```python
from build123d import *
from build123d.topology import SkipClean

# Parameters (mm, degrees)
SKETCH1_W             = 80
SKETCH1_H             = 80
BOSS_EXTRUDE1_DEPTH   = 1.5
FILLET1_R             = 4
BOSS_EXTRUDE2_START   = 1.5
SKETCH2_R             = 4
BOSS_EXTRUDE2_DEPTH   = 1.5
F_4_0MM_DOWEL_HOLE1_D = 4
CUT_EXTRUDE1_DEPTH    = 1.5


with BuildPart() as part:
    # Sketch1 → Boss-Extrude1 (new body)
    with BuildSketch(Plane.XY):
        with Locations((40, 40)):
            Rectangle(SKETCH1_W, SKETCH1_H)
    extrude(amount=BOSS_EXTRUDE1_DEPTH)

    # Fillet1
    fillet1_edges = [part.edges().sort_by_distance(p)[0] for p in [
        (0, 0, 0.75),
        (0, 80, 0.75),
        (80, 80, 0.75),
        (80, 0, 0.75),
    ]]
    fillet(fillet1_edges, radius=FILLET1_R)

    # Sketch2 → Boss-Extrude2 (add)
    with SkipClean():  # the faces are left unmerged after this step: merging them gives an invalid solid
        with BuildSketch(Plane.XY.offset(1.5).offset(BOSS_EXTRUDE2_START)):
            with Locations(Location((4, 76, 0), (0, 0, 180))):
                Circle(SKETCH2_R)
            with Locations((76, 76)):
                Circle(SKETCH2_R)
            with Locations((4, 4)):
                Circle(SKETCH2_R)
            with Locations((76, 4)):
                Circle(SKETCH2_R)
        extrude(amount=-BOSS_EXTRUDE2_DEPTH)

    # 4.0mm Dowel Hole1 (through all)
    with Locations(Plane(origin=(0, 0, 0), x_dir=(-1, 0, 0), z_dir=(0, 0, -1))):
        with Locations((-4, 4), (-76, 4), (-76, 76), (-4, 76)):
            Hole(F_4_0MM_DOWEL_HOLE1_D / 2)

    # Sketch5 → Cut-Extrude1 (cut)
    with SkipClean():  # the faces are left unmerged after this step: merging them gives an invalid solid
        with BuildSketch(Plane(origin=(0, 0, 0), x_dir=(-1, 0, 0), z_dir=(0, 0, -1))):
            with BuildLine():
                Line((-55.934284639, 54.434284639), (-71, 69.5))
                Line((-71, 69.5), (-71, 10.5))
                Line((-71, 10.5), (-55.934284639, 25.565715361))
                ThreePointArc((-55.934284639, 25.565715361), (-61.5, 40), (-55.934284639, 54.434284639))
            make_face()
            with BuildLine():
                Line((-41.5, 40), (-54.164078425, 52.664078425))
                ThreePointArc((-54.164078425, 52.664078425), (-59, 40), (-54.164078425, 27.335921575))
                Line((-54.164078425, 27.335921575), (-41.5, 40))
            make_face()
            with BuildLine():
                Line((-40, 41.5), (-27.335921575, 54.164078425))
                ThreePointArc((-27.335921575, 54.164078425), (-40, 59), (-52.664078425, 54.164078425))
                Line((-52.664078425, 54.164078425), (-40, 41.5))
            make_face()
            with BuildLine():
                Line((-10.5, 71), (-69.5, 71))
                Line((-69.5, 71), (-54.434284639, 55.934284639))
                ThreePointArc((-54.434284639, 55.934284639), (-40, 61.5), (-25.565715361, 55.934284639))
                Line((-25.565715361, 55.934284639), (-10.5, 71))
            make_face()
            with BuildLine():
                Line((-9, 10.5), (-9, 69.5))
                Line((-9, 69.5), (-24.065715361, 54.434284639))
                ThreePointArc((-24.065715361, 54.434284639), (-18.5, 40), (-24.065715361, 25.565715361))
                Line((-24.065715361, 25.565715361), (-9, 10.5))
            make_face()
            with BuildLine():
                Line((-25.835921575, 27.335921575), (-38.5, 40))
                Line((-38.5, 40), (-25.835921575, 52.664078425))
                ThreePointArc((-25.835921575, 52.664078425), (-21, 40), (-25.835921575, 27.335921575))
            make_face()
            with BuildLine():
                Line((-52.664078425, 25.835921575), (-40, 38.5))
                Line((-40, 38.5), (-27.335921575, 25.835921575))
                ThreePointArc((-27.335921575, 25.835921575), (-40, 21), (-52.664078425, 25.835921575))
            make_face()
            with BuildLine():
                Line((-54.434284639, 24.065715361), (-69.5, 9))
                Line((-69.5, 9), (-10.5, 9))
                Line((-10.5, 9), (-25.565715361, 24.065715361))
                ThreePointArc((-25.565715361, 24.065715361), (-40, 18.5), (-54.434284639, 24.065715361))
            make_face()
        extrude(amount=-CUT_EXTRUDE1_DEPTH, mode=Mode.SUBTRACT)
    add(part.part.scale(1), mode=Mode.REPLACE)  # the faces are merged on a copy


solid = part.part
```
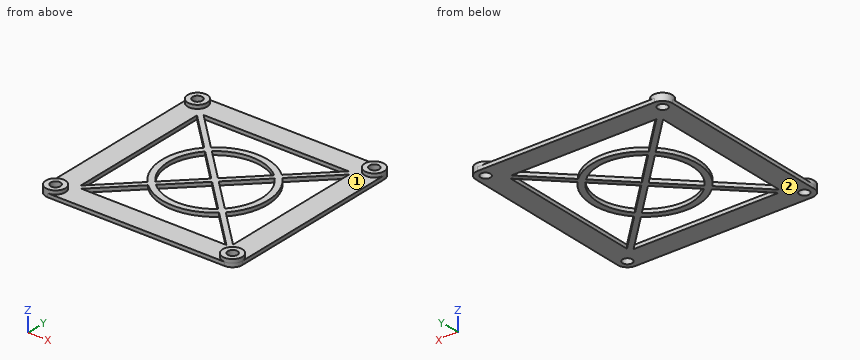
Geometry: final body of the model. Coordinates: model frame, mm. Face numbers are marked on the shaded views. Coordinates: 2 decimals unless noted, no trailing zeros. Write each loop counter-clockwise with the first axis right and the second up, starting at its lowest first coordinate (ties: lowest second). Pieces come first, ordered by that corner, then holes. Notation, with made-up numbers: M 55,69.25 L 89,69.25 A15 ccw 89,82.25 Z; hole C -6.5,86 d4. An arc over 180 degrees is marked long. Use CSV: the item, a comma, the result in double quotes. Start each with the question number.
1. First-contact query: P1, Ø24, axis at x = 26, y = 23.5, coming from the +Z side. Flat tip, straight axial feed; report the tip coordinate or a pass-through.
2. Ray query, probe 1 along Y at (x, z) = (4, 2.1); probe 2 along Y at (x, z) = (74.5, 0.45); probe 3 along Y at (x, z) = (76, 0.95). Return the intervals inside material, ascending.
3. Cut plane B-B on y = 64.5. Return the cut outline in (x, z), plus the area to 3 significant figures.
4. Cut plane D-D on x = 44.5. Return the cut outline in (y, z).
5. Mould query, pull axis Y, two halves, no side actions, for the marked faces 1 and 2. Classes: pulls with the +Y half, pulls with the -Y half, needs draft (parallel to the pull), parting line crosses it, or undercut.
6. Cut plane A-A on x = 66.5. Return the cut outline in (y, z).
7. Cut plane C-C on z = 0.6. Count the separate pieces of the cut face and the enclosed holes in it, plus the area to 3 significant figures.
Entries:
1,P1,"z = 1.5"
2,probe 1,"0 to 2, 6 to 8, 72 to 74, 78 to 80"
2,probe 2,"0 to 2.68, 5.32 to 74.68, 77.32 to 80"
2,probe 3,"0 to 2, 6 to 74, 78 to 80"
3,outline,"M 0,0 L 9,0 L 9,1.5 L 0,1.5 Z; M 14,0 L 17,0 L 17,1.5 L 14,1.5 Z; M 63,0 L 66,0 L 66,1.5 L 63,1.5 Z; M 71,0 L 80,0 L 80,1.5 L 71,1.5 Z"
3,area,"36.0 mm²"
4,outline,"M 0,0 L 9,0 L 9,1.5 L 0,1.5 Z; M 18.98,0 L 21.54,0 L 21.54,1.5 L 18.98,1.5 Z; M 34,0 L 37,0 L 37,1.5 L 34,1.5 Z; M 43,0 L 46,0 L 46,1.5 L 43,1.5 Z; M 58.46,0 L 61.02,0 L 61.02,1.5 L 58.46,1.5 Z; M 71,0 L 80,0 L 80,1.5 L 71,1.5 Z"
5,face 1,"undercut"
5,face 2,"needs draft"
6,outline,"M 0,0 L 9,0 L 9,1.5 L 0,1.5 Z; M 12,0 L 15,0 L 15,1.5 L 12,1.5 Z; M 65,0 L 68,0 L 68,1.5 L 65,1.5 Z; M 71,0 L 80,0 L 80,1.5 L 71,1.5 Z"
7,separate pieces,"1"
7,enclosed holes,"12"
7,area,"3,150 mm²"
